Source: CAD feature listing. Evaluate the final solid. Frame: model axes, mm. A direction names the side the tool comes from. Give positions to 0.01 mm unless a question says otherwise; leave off trailing zeros. Order: outer loops, then holes, each group sorted by start corner. A loop starts at its lowest first (then second) coordinate and runs counter-clockwise, first axis right, second up.
1) Section C-C, the plane z = 39.25. Return loops of the section in (x, y).
2) First-contact query: P1, Ø1, axis at x = 49, z = 40.5, coming from the -Y side; P2, Ø1.5, axis at y = 6.5, z = 41, coming from the +X side. Flat tips, straight axial feed; report the tip coordinate or a pass-through.
3) Section B-B, the plane x = 51.05. Return loops of the section in (y, z), plus the area to 3 significant figures.
4) Material intervals for line 1 (Z direction, x = 51.75, y = 8.45); line 2 (Y direction, x = 50.2, z = 40.1); line 3 (X direction, y = 7.1, z = 39.05), sorted ascending.
5) Access query for faces 1 (the face through (50, 5, 39)), 2 (the face through (52.31, 6.04, 38.49)). Directions: +Z, -Z, +X, -X, +Y, -Y. A direction counts if a zero-diameter tool reaches every point of the face in a straight line with its end or side. Return the directions, or none.
6) Section A-A, the plane y = 7. Return loops of the section in (x, z), plus the area to 3 significant figures.
7) Section D-D, the plane z = 38.7. Return loops of the section in (x, y).
```python
from build123d import *

# Parameters (mm, degrees)
CYLINDER014_R     = 2.5
CYLINDER014_DEPTH = 1
CYLINDER013_R     = 1.5
CYLINDER013_DEPTH = 5


with BuildPart() as button_base:
    # Cylinder014 → Cylinder014 (new body)
    with BuildSketch(Plane(origin=(50, 7, 37), x_dir=(1, 0, 0), z_dir=(0, 0, 1))):
        Circle(CYLINDER014_R)
    extrude(amount=CYLINDER014_DEPTH)


with BuildPart() as button001:
    # Cylinder013 → Cylinder013 (new body)
    with BuildSketch(Plane(origin=(50, 7, 37), x_dir=(1, 0, 0), z_dir=(0, 0, 1))):
        Circle(CYLINDER013_R)
    extrude(amount=CYLINDER013_DEPTH)

    # Fusion009: union button_base
    add(button_base.part)


with BuildPart() as button001_1:
    # Fusion009 placement: moved
    add(button001.part.moved(Location((0, 0, 1))))


solid = button001_1.part
```
From the geometry:
1. outline: circle Ø3 at (50, 7)
2. P1: stops at y = 5.59
2. P2: stops at x = 51.5
3. outline: (4.73, 38) - (9.27, 38) - (9.27, 39) - (8.07, 39) - (8.07, 43) - (5.93, 43) - (5.93, 39) - (4.73, 39) - close
3. area: 13.1 mm2
4. line 1: z = 38 to 39
4. line 2: y = 5.51 to 8.49
4. line 3: x = 48.5 to 51.5
5. face 1: +Z
5. face 2: +Z, -Z
6. outline: (47.5, 38) - (52.5, 38) - (52.5, 39) - (51.5, 39) - (51.5, 43) - (48.5, 43) - (48.5, 39) - (47.5, 39) - close
6. area: 17.0 mm2
7. outline: circle Ø5 at (50, 7)
